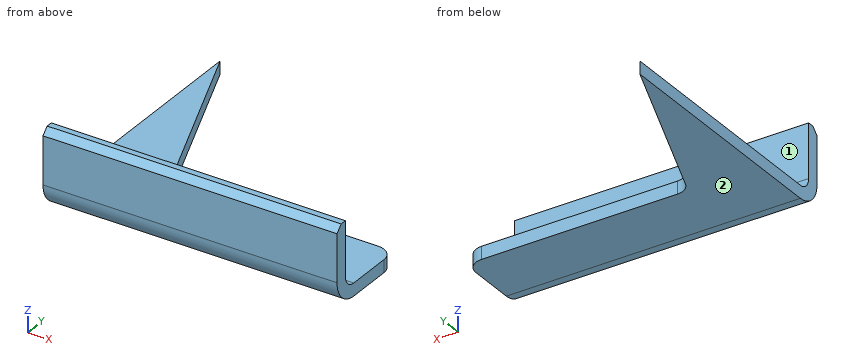
```python
from build123d import *

# Parameters (mm, degrees)
SM_BASE_FLANGE_1_DEPTH           = 8
SM_EDGE_FLANGE_1_STRIP_W         = 48
SM_EDGE_FLANGE_1_STRIP_H         = 8
SM_EDGE_FLANGE_1_STRIP_CUT_DEPTH = 185
SM_EDGE_FLANGE_1_DEPTH           = 185
FILLET_1_R                       = 10
CHAMFER_1_SIZE                   = 4


# Sheet-metal steps are written as plain solids
with BuildPart() as part:
    # Sketch 1 → 基体-法兰1 (new body)
    with BuildSketch(Plane.XY):
        Polygon((0, 0), (45, -115), (185, -115), (185, -170), (0, -170), align=None)
    extrude(amount=-SM_BASE_FLANGE_1_DEPTH)

    # 边线-法兰1 strip (across the edge) → 边线-法兰1 strip cut (cut)
    with BuildSketch(Plane(origin=(0, -170, 0), x_dir=(0, 1, 0), z_dir=(1, 0, 0))):
        with Locations((-8, -4)):
            Rectangle(SM_EDGE_FLANGE_1_STRIP_W, SM_EDGE_FLANGE_1_STRIP_H)
    extrude(amount=SM_EDGE_FLANGE_1_STRIP_CUT_DEPTH, mode=Mode.SUBTRACT)

    # 边线-法兰1 section (across the edge) → 边线-法兰1 (add)
    with BuildSketch(Plane(origin=(0, -170, 0), x_dir=(0, 1, 0), z_dir=(1, 0, 0))):
        with BuildLine():
            Line((0, 8), (0, 42))
            Line((0, 42), (8, 42))
            Line((8, 42), (8, 8))
            ThreePointArc((8, 8), (10.343145751, 2.343145751), (16, 0))
            Line((16, 0), (16, -8))
            ThreePointArc((16, -8), (4.686291501, -3.313708499), (0, 8))
        make_face()
    extrude(amount=SM_EDGE_FLANGE_1_DEPTH)

    # 圆角1
    fillet_1_edges = [part.edges().sort_by_distance(p)[0] for p in [
        (45, -115, -4),
        (185, -115, -4),
    ]]
    fillet(fillet_1_edges, radius=FILLET_1_R)

    # 倒角1
    chamfer_1_edges = [part.edges().sort_by_distance(p)[0] for p in [
        (92.5, -170, 42),
    ]]
    chamfer(chamfer_1_edges, length=CHAMFER_1_SIZE)


solid = part.part
```
Here's how the part is built. I have some questions about the finished solid (model axes, mm). Face numbers are marked on the shaded views. A direction names the side the tool comes from. Round coordinates to 2 decimals unless told otherwise and drop trailing zeros. Write each loop counter-clockwise with the first axis right and the second up, starting at its lowest first coordinate (ties: lowest second). Pieces come first, ordered by that corner, then holes.
Q1. If we section it at B-B on z = -4.5: Write out the boundary of the cut face in (x, y), plus the area to 3 significant figures.
Q2. Which directions (+Z, -Z, +X, -X, +Y, -Y) give clear straight access to the entire face, cutting with the end or side of a thin tool? Please do the marked faces 1 and 2.
Q3. If we section it at A-A on x = 62: Write out the boundary of the cut face in (y, z), plus the area to 3 significant figures.
Q4. If we section it at D-D on z = 33: Write out the boundary of the cut face in (x, y), plus the area to 3 significant figures.
Q5. Will these pins go through, and if not, where does the flat tip stop? P1, Ø3, axis at x = 58.5, z = 4.5, coming from the -Y side; P2, Ø9, axis at x = 95.5, z = -5.5, coming from the +Y side; P3, Ø12, axis at x = 86, z = 31, coming from the +Y side; P4, Ø10, axis at y = -122.5, z = -2, coming from the +X side.
Q6. If we section it at C-C on y = -79.5: Write out the boundary of the cut face in (x, z), plus the area to 3 significant figures.
Q7. Please list where these lines run through material, in increasing order: probe 1 along Y at (x, z) = (129.5, 15.5); probe 2 along Z at (x, y) = (87, -150); probe 3 along Z at (x, y) = (96, -156.5).
Answer below:
1. outline: (0, -163.99) - (185, -163.99) - (185, -125) arc R10 ccw to (175, -115) - (51.83, -115) arc R10 cw to (42.51, -108.64) - (0, 0) - close
1. area: 11,600 mm2
2. face 1: +Z, +X, -X, +Y
2. face 2: -Z, +X, -X, +Y, -Y
3. outline: (-170, 8) arc R16 ccw to (-154, -8) - (-115, -8) - (-115, 0) - (-154, 0) arc R8 cw to (-162, 8) - (-162, 42) - (-166, 42) - (-170, 38) - close
3. area: 727 mm2
4. outline: (0, -170) - (185, -170) - (185, -162) - (0, -162) - close
4. area: 1,480 mm2
5. P1: stops at y = -169.87
5. P2: stops at y = -115
5. P3: stops at y = -162
5. P4: stops at x = 185
6. outline: (0, -8) - (31.11, -8) - (31.11, 0) - (0, 0) - close
6. area: 249 mm2
7. probe 1: y = -170 to -162
7. probe 2: z = -8 to 0
7. probe 3: z = -7.8 to 0.4
